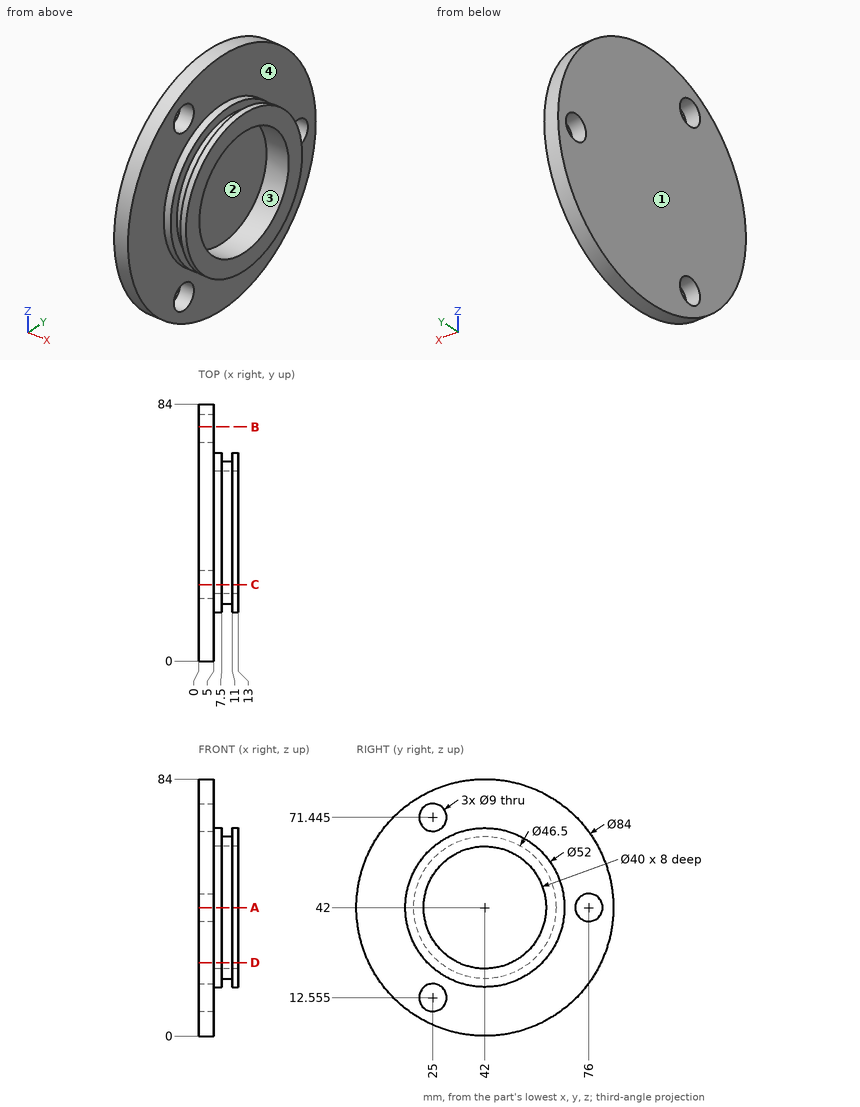
Could you check a few things on this drawing? It's one solid part, dimensions in mm from its lowest x, y, z. A direction names the side the tool comes from. Coordinates: 2 decimals unless noted, no trailing zeros. Loops run counter-clockwise (first coordinate to the right, second up) from the corner with the lowest first, then second, coordinate; pieces in that order, holes last.
1. Imagine slicing it at A-A (z = 42). Please give me the cut outline in (x, y), and give its area (3 significant figures).
2. For P1, Ø5, axis at y = 48, z = 14, coming from the +X side; P2, Ø3, axis at x = 7.5, z = 26.5, coming from the +Y side; P3, Ø3, axis at x = 5, y = 18.5, coming from the +Z side, each with a flat end and sliding along its axis, tell me the tip position at first contact or that it passes through.
3. Imagine slicing it at B-B (y = 76.5). Please give me the cut outline in (x, z), and give its area (3 significant figures).
4. Imagine slicing it at C-C (y = 25). Please give me the cut outline in (x, z) (1 decimal), and give its area (3 significant figures).
5. Imagine slicing it at D-D (z = 24). Please give me the cut outline in (x, y), and give its area (3 significant figures).
6. I need wall thicknesses on L1, parallel to Z at x = 2.2, y = 25 (1 decimal); L2, parallel to Z at x = 11.75, y = 42; L3, parallel to Z at x = 8.5, y = 42. Which ranges of each line are inside material? Lowest first, please.
7. For the marked faces 1 and 2, which set-ups out of +Z, -Z, +X, -X, +Y, -Y let a thin tool reach every point of the face, with its end or its side?
8. We'd pull the mould along Y, two halves only. Please class the marked faces 3 and 4: released by +Y, released by -Y, zero draft, split by the parting line, or undercut.
Computed values:
1. outline: (0, 0) - (5, 0) - (5, 16) - (7.5, 16) - (7.5, 18.75) - (11, 18.75) - (11, 16) - (13, 16) - (13, 22) - (5, 22) - (5, 62) - (13, 62) - (13, 68) - (11, 68) - (11, 65.25) - (7.5, 65.25) - (7.5, 68) - (5, 68) - (5, 71.5) - (0, 71.5) - close; (0, 80.5) - (5, 80.5) - (5, 84) - (0, 84) - close
1. area: 452 mm2
2. P1: stops at x = 5
2. P2: stops at y = 63.91
2. P3: stops at z = 77.78
3. outline: (0, 18.05) - (5, 18.05) - (5, 37.53) - (0, 37.53) - close; (0, 46.47) - (5, 46.47) - (5, 65.95) - (0, 65.95) - close
3. area: 195 mm2
4. outline: (0, 3.6) - (5, 3.6) - (5, 8.1) - (0, 8.1) - close; (0, 17.1) - (5, 17.1) - (5, 22.3) - (7.5, 22.3) - (7.5, 26.1) - (11, 26.1) - (11, 22.3) - (13, 22.3) - (13, 31.5) - (5, 31.5) - (5, 52.5) - (13, 52.5) - (13, 61.7) - (11, 61.7) - (11, 57.9) - (7.5, 57.9) - (7.5, 61.7) - (5, 61.7) - (5, 66.9) - (0, 66.9) - close; (0, 75.9) - (5, 75.9) - (5, 80.4) - (0, 80.4) - close
4. area: 414 mm2
5. outline: (0, 4.05) - (5, 4.05) - (5, 23.24) - (7.5, 23.24) - (7.5, 27.28) - (11, 27.28) - (11, 23.24) - (13, 23.24) - (13, 33.28) - (5, 33.28) - (5, 50.72) - (13, 50.72) - (13, 60.76) - (11, 60.76) - (11, 56.72) - (7.5, 56.72) - (7.5, 60.76) - (5, 60.76) - (5, 79.95) - (0, 79.95) - close
5. area: 512 mm2
6. L1: z = 3.6 to 8.1, 17.1 to 66.9, 75.9 to 80.4
6. L2: z = 16 to 22, 62 to 68
6. L3: z = 18.75 to 22, 62 to 65.25
7. face 1: +Z, -Z, -X, +Y, -Y
7. face 2: +X
8. face 3: undercut
8. face 4: zero draft
